Autodesk Inventor part; units mm, degrees
ref_plane "YZ Plane" through (0, 0, 0) normal (1, 0, 0) x (0, 1, 0)
ref_plane "XZ Plane" through (0, 0, 0) normal (0, 1, 0) x (-1, 0, 0)
ref_plane "XY Plane" through (0, 0, 0) normal (0, 0, 1) x (1, 0, 0)
sketch "Skizze1" plane through (0, 0, 0) normal (0, 1, 0) x (-1, 0, 0)
  line L0 (-96.0755, -26.209) -> (-136.0755, -26.209)
  line L1 (-136.0755, -26.209) -> (-136.0755, -56.209)
  line L2 (-136.0755, -56.209) -> (-96.0755, -56.209)
  line L3 (-96.0755, -56.209) -> (-96.0755, -26.209)
  point P0 (0, 0)
  dimension "d0" = 40
  dimension "d1" = 30
extrude "Extrusion1" add sketch "Skizze1" along normal blind 42
sketch "Skizze4" plane through (96.0755, 0, -26.209) normal (0, 0, 1) x (1, 0, 0)
  line L0 (0, 0) -> (40, 0)
  line L1 (40, 0) -> (40, 42)
  line L2 (0, 42) -> (40, 42)
  line L3 (0, 0) -> (0, 42)
  line L4 (0, 0) -> (40, 0)
  line L5 (40, 0) -> (40, 42)
  line L6 (0, 42) -> (40, 42)
  line L7 (0, 0) -> (0, 42)
  circle A0 centre (20, 21) radius 3.7853
  point P0 (-96.0755, 0)
extrude "Extrusion3" cut sketch "Skizze4" against normal blind 10 contours A0
sketch "Skizze3" plane through (0, 42, 0) normal (0, 1, 0) x (1, 0, 0)
  circle A0 centre (130.0755, 50.209) radius 1.5
  circle A1 centre (111.5755, 50.209) radius 1.5
  circle A2 centre (116.0755, 31.709) radius 1.5
  line L0 (136.0755, 56.209) -> (96.0755, 56.209)
  line L1 (136.0755, 26.209) -> (136.0755, 56.209)
  point P0 (0, 0)
  dimension "d4" = 3
  dimension "d5" = 3
  dimension "d6" = 3
  dimension "d7" = 6
  dimension "d8" = 6
  dimension "d9" = 6
  dimension "d10" = 18.5
  dimension "d11" = 18.5
  dimension "d12" = 20
extrude "Extrusion2" cut sketch "Skizze3" against normal blind 10
pattern_circular "Runde Anordnung1" count 2 over 360 about axis through (116.0755, 21, -26.209) along (0, 0, -1) of "Extrusion2"
properties part number "01_Coolingblock"
The listing builds one solid part. Answer for the finished solid, in the listing's coordinates (mm). A direction names the side the tool comes from. Coordinates: 2 decimals unless noted, no trailing zeros. Loops run counter-clockwise (first coordinate to the right, second up) from the corner with the lowest first, then second, coordinate; pieces in that order, holes last. Notation, with made-up numbers: (-40, 79.5) -> (-28, 79.5) arc R18 ccw to (-28, 108.5) -> close; hole circle Ø10 at (68, 40.5). An arc over 180 degrees is marked (long way). Return JSON: item names as keys, results as strings. Group by question number.
(1) A cutting plane is placed at A-A on y = 21. Write down the section's boundary in (x, z), and give its area (3 significant figures).
(2) Given pin 1 Ø0.9 at (x, z) = (130.5, -51) entering from +Y; pin 2 Ø1.5 at (x, z) = (102.5, -50.5) entering from -Y, each flat-ended and moving along its own axis, determine where each tip first touches the part or whether it passes through.
(3) A cutting plane is placed at B-B on z = -31. Write down the section's boundary in (x, y).
(4) Which of the six approach directions +Z, -Z, +X, -X, +Y, -Y give full straight-line access (tool end or side, diameter ignored) to faces 1 (the flat face through (112, 32, -50)), 2 (the flat face through (116, 21, -56.209)), 3 (the cylindrical face through (119.57, 19.55, -31.14)), 4 (the flat face through (116, 0, -41)), 5 (the cylindrical face through (116.401, 4.93, -30.245))?
(5) A cutting plane is placed at C-C on z = -49.5. Write down the section's boundary in (x, y).
(6) A cutting plane is placed at D-D on y = 39. Write down the section's boundary in (x, z), and give its area (3 significant figures).
(7) Find the intervals of material crossed by probe 1 along X at (y, z) = (35.5, -49.5); probe 2 along Z at (x, y) = (117, 34), in increasing order. Write a range as from..to.
(8) Determine the mould class of faces 6 (the flat face through (116, 42, -41)), 7 (the cylindrical face through (101.38, 4.93, -48.88)), 8 (the flat face through (136.076, 21, -41)) for opening direction X: released by +X, released by -X, zero draft, split by the parting line, or undercut.
The answers:
{
 "1": {"outline": "(96.08, -56.21) -> (136.08, -56.21) -> (136.08, -26.21) -> (119.86, -26.21) -> (119.86, -36.21) -> (112.29, -36.21) -> (112.29, -26.21) -> (96.08, -26.21) -> close", "area": "1,120 mm^2"},
 "2": {"pin 1": "stops at y = 32", "pin 2": "stops at y = 10"},
 "3": {"outline": "(96.08, 0) -> (114.75, 0) -> (114.75, 10) -> (117.4, 10) -> (117.4, 0) -> (136.08, 0) -> (136.08, 42) -> (117.4, 42) -> (117.4, 32) -> (114.75, 32) -> (114.75, 42) -> (96.08, 42) -> close; hole circle Ø7.57 at (116.08, 21)"},
 "4": {"face 1": "+Y", "face 2": "-Z, +X, -X, +Y, -Y", "face 3": "+Z", "face 4": "+Z, -Z, +X, -X, -Y", "face 5": "-Y"},
 "5": {"outline": "(96.08, 0) -> (100.75, 0) -> (100.75, 10) -> (103.4, 10) -> (103.4, 0) -> (119.25, 0) -> (119.25, 10) -> (121.9, 10) -> (121.9, 0) -> (136.08, 0) -> (136.08, 42) -> (131.4, 42) -> (131.4, 32) -> (128.75, 32) -> (128.75, 42) -> (112.9, 42) -> (112.9, 32) -> (110.25, 32) -> (110.25, 42) -> (96.08, 42) -> close"},
 "6": {"outline": "(96.08, -56.21) -> (136.08, -56.21) -> (136.08, -26.21) -> (96.08, -26.21) -> close; hole circle Ø3 at (111.58, -50.21); hole circle Ø3 at (116.08, -31.71); hole circle Ø3 at (130.08, -50.21)", "area": "1,180 mm^2"},
 "7": {"probe 1": "x = 96.08..110.25, 112.9..128.75, 131.4..136.08", "probe 2": "z = -56.21..-32.89, -30.53..-26.21"},
 "8": {"face 6": "zero draft", "face 7": "undercut", "face 8": "released by +X"}
}
